The listing builds one solid part. Answer for the finished solid, in the listing's coordinates (mm). Round coordinates to 2 decimals unless told otherwise and drop trailing zeros. Loops run counter-clockwise (first coordinate to the right, second up) from the corner with the lowest first, then second, coordinate; pieces in that order, holes last. Notation, with made-up numbers: (66, 61.5) -> (87, 61.5) arc R25 cw to (87, 100.5) -> close; hole circle Ø6 at (88.5, 72.5). An arc over 180 degrees is marked (long way). Write each question's results on one line, items separated by ' | '. Start each with the question number.
(1) The part is cut by section A-A (x = 12). Determine the outline of the cut face in (y, z), plus the area to 3 significant figures.
(2) The part is cut by section C-C (y = 20). Determine the outline of the cut face in (x, z), plus the area to 3 significant figures.
(3) A flat-ended cylindrical pin translates along its axis: pin 1 (4 mm diameter, centred on y = 23.5, z = 5.5, fed in from -X). Find the tip coordinate at first contact, or state that the pin passes through.
(4) The part is cut by section D-D (x = 25). Determine the outline of the cut face in (y, z).
(5) Determine the mould class of faces 1 (the face through (30, 6, 3)), 2 (the face through (0, 6, 3)), 3 (the face through (11.826, 14.052, 3.448)) for opening direction X: released by +X, released by -X, zero draft, split by the parting line, or undercut.
(6) Straight lines are drawn through the part: probe 1 along Y at (x, z) = (15, 4); probe 2 along X at (y, z) = (19.5, 1.75); probe 3 along Y at (x, z) = (17.5, 4). For each, find the intervals that lie inside material, in ascending order.
```python
from build123d import *

# Parameters (mm, degrees)
CROQUIS1_W              = 30
CROQUIS1_H              = 26.322580645
SALIENTE_EXTRUIR1_DEPTH = 6.8
REDONDEO1_R             = 15
CORTAR_EXTRUIR1_REACH   = 42.486
CROQUIS2_R              = 4


with BuildPart() as part:
    # Croquis1 → Saliente-Extruir1 (new body)
    with BuildSketch(Plane.XY):
        with Locations((15, 13.161290323)):
            Rectangle(CROQUIS1_W, CROQUIS1_H)
    extrude(amount=SALIENTE_EXTRUIR1_DEPTH)

    # Redondeo1
    redondeo1_edges = [part.edges().sort_by_distance(p)[0] for p in [
        (0, 26.322580645, 3.4),
        (30, 26.322580645, 3.4),
    ]]
    fillet(redondeo1_edges, radius=REDONDEO1_R - 0.0001)  # a hair under: the kernel refuses the full size

    # Croquis2 → Cortar-Extruir1 (cut, up to next)
    with BuildSketch(Plane.XY.offset(6.8), mode=Mode.PRIVATE) as cortar_extruir1_sk1:
        with Locations((15, 16.485572524)):
            Circle(CROQUIS2_R)
    cortar_extruir1_tool1 = extrude(cortar_extruir1_sk1.sketch, amount=-CORTAR_EXTRUIR1_REACH, mode=Mode.PRIVATE) & part.part
    add(cortar_extruir1_tool1.solids().sort_by_distance((15, 16.485573, 6.8))[0], mode=Mode.SUBTRACT)


solid = part.part
```
Checked values:
1) outline: (0, 0) -> (13.84, 0) -> (13.84, 6.8) -> (0, 6.8) -> close; (19.13, 0) -> (26.02, 0) -> (26.02, 6.8) -> (19.13, 6.8) -> close | area: 141 mm2
2) outline: (2.76, 0) -> (13.09, 0) -> (13.09, 6.8) -> (2.76, 6.8) -> close; (16.91, 0) -> (27.24, 0) -> (27.24, 6.8) -> (16.91, 6.8) -> close | area: 140 mm2
3) pin 1: stops at x = 3.98
4) outline: (0, 0) -> (22.5, 0) -> (22.5, 6.8) -> (0, 6.8) -> close
5) face 1: released by +X | face 2: released by -X | face 3: undercut
6) probe 1: y = 0 to 12.49, 20.49 to 26.32 | probe 2: x = 2.42 to 12.37, 17.63 to 27.58 | probe 3: y = 0 to 13.36, 19.61 to 26.11
